```python
from build123d import *

# Parameters (mm, degrees)
CUT_EXTRUDE1_START = -1.5
CUT_EXTRUDE1_DEPTH = 1.5
SKETCH4_R          = 1.443375673
CUT_EXTRUDE2_DEPTH = 0.5
CUT_EXTRUDE2_DRAFT = -45


with BuildPart() as part:
    # Sketch2 → Revolve1 (revolve)
    with BuildSketch(Plane(origin=(0, 0, 0), x_dir=(0, 0, -1), z_dir=(1, 0, 0)), mode=Mode.PRIVATE) as revolve1_sk:
        Polygon((-8.35, 2.75), (-5.65, 2.75), (-5.5, 2.6), (-5.5, 1.5), (8, 1.5), (8.5, 1), (8.5, 0), (-8.5, 0), (-8.5, 2.6), align=None)
    revolve(revolve1_sk.sketch.rotate(Axis((0, 0, -8.5), (0, 0, 1)), 90), axis=Axis((0, 0, -8.5), (0, 0, 1)))

    # Sketch3 → Cut-Extrude1 (cut)
    with BuildSketch(Plane.XY.offset(8.5).offset(CUT_EXTRUDE1_START)):
        Polygon((0, 1.443375673), (-1.25, 0.721687836), (-1.25, -0.721687836), (0, -1.443375673), (1.25, -0.721687836), (1.25, 0.721687836), align=None)
    extrude(amount=CUT_EXTRUDE1_DEPTH, mode=Mode.SUBTRACT)


with BuildPart() as cut_extrude2_tool:
    # Sketch4 → Cut-Extrude2 (with draft: the straight prism first)
    with BuildSketch(Plane.XY.offset(8.5)):
        Circle(SKETCH4_R)
    extrude(amount=-CUT_EXTRUDE2_DEPTH)
    # Cut-Extrude2: the draft: its side faces are tilted about the plane it starts from
    cut_extrude2_sides = [cut_extrude2_tool.faces().sort_by_distance(p)[0] for p in [
        (-1.443375673, 0, 8.25),
    ]]
    draft(cut_extrude2_sides, Plane.XY.offset(8.5), CUT_EXTRUDE2_DRAFT)


with BuildPart() as part_1:
    add(part.part)

    # Cut-Extrude2: cut by cut_extrude2_tool
    add(cut_extrude2_tool.part, mode=Mode.SUBTRACT)


solid = part_1.part
```
Read the model definition and answer for the solid it produces. Units are mm, in the model's axes. A direction names the side the tool comes from. Round coordinates to 2 decimals unless told otherwise and drop trailing zeros. Write each loop counter-clockwise with the first axis right and the second up, starting at its lowest first coordinate (ties: lowest second). Pieces come first, ordered by that corner, then holes. Notation, with made-up numbers: M 66,-9 L 102,-9 A22 ccw 102,11 Z; hole C 32,-35 d6. An arc over 180 degrees is marked long. One line per item, written item: value.
Q1. Which of the six approach directions +Z, -Z, +X, -X, +Y, -Y give full straight-line access (tool end or side, diameter ignored) to faces 4 (the flat face through (0.63, 1.08, 7.74)), 5 (the flat face through (0, 2, 5.5)), 6 (the flat face through (0, 2, 8.5))?
Data:
face 4: +Z
face 5: -Z
face 6: +Z, +X, -X, +Y, -Y
Q2. Straight lines are drawn through the part: line 1 (Z direction, x = 0.7, y = -1.4); line 2 (Y direction, x = 1.2, z = 2.75); line 3 (X direction, y = 0.2, z = 2.5). For each, find the intervals that lie inside material, in ascending order. Write a range as [from, to].
Data:
line 1: [5.5, 8.5]
line 2: [-0.9, 0.9]
line 3: [-1.49, 1.49]
Q3. Flat-ended cylindrical pins translate along their axes: pin 1 Ø2 at (x, y) = (-0.5, 1) entering from +Z; pin 2 Ø2 at (x, z) = (1, 5) entering from -Y; pin 3 Ø0.8 at (x, y) = (0.5, 0.5) entering from +Z; pin 4 Ø1.5 at (y, z) = (-0.5, 1.5) entering from -X. Find the tip coordinate at first contact, or state that the pin passes through.
Data:
pin 1: z = 8.5
pin 2: y = -2.74
pin 3: z = 7
pin 4: x = -1.5
Q4. Find section A-A on z = 7.75. Write down the section's boundary in (x, y).
Data:
outline: C 0,0 d5.5; hole M -1.25,-0.72 L 0,-1.44 L 1.25,-0.72 L 1.25,0.72 L 0,1.44 L -1.25,0.72 Z
Q5. Find section C-C on z = -7. Write down the section's boundary in (x, y).
Data:
outline: C 0,0 d3
Q6. For a pull along Y with two mould halves and no side action, classify faces 1 (the cylindrical face through (0.596, 2.685, 6.981)), 2 (the flat face through (0, 0, -8.5)), 3 (the flat face through (-1.25, 0, 8)) as +Y half, -Y half, draft (parallel to the pull), parting line (faces both ways), or undercut.
Data:
face 1: parting line
face 2: draft
face 3: undercut
Q7. Find section B-B on y = 0. Write down the section's boundary in (x, z), plus the area to 3 significant figures.
Data:
outline: M -2.75,5.65 L -2.6,5.5 L -1.5,5.5 L -1.5,-8 L -1,-8.5 L 1,-8.5 L 1.5,-8 L 1.5,5.5 L 2.6,5.5 L 2.75,5.65 L 2.75,8.35 L 2.6,8.5 L 1.44,8.5 L 1.25,8.31 L 1.25,7 L -1.25,7 L -1.25,8.31 L -1.44,8.5 L -2.6,8.5 L -2.75,8.35 Z
area: 54.4 mm2
